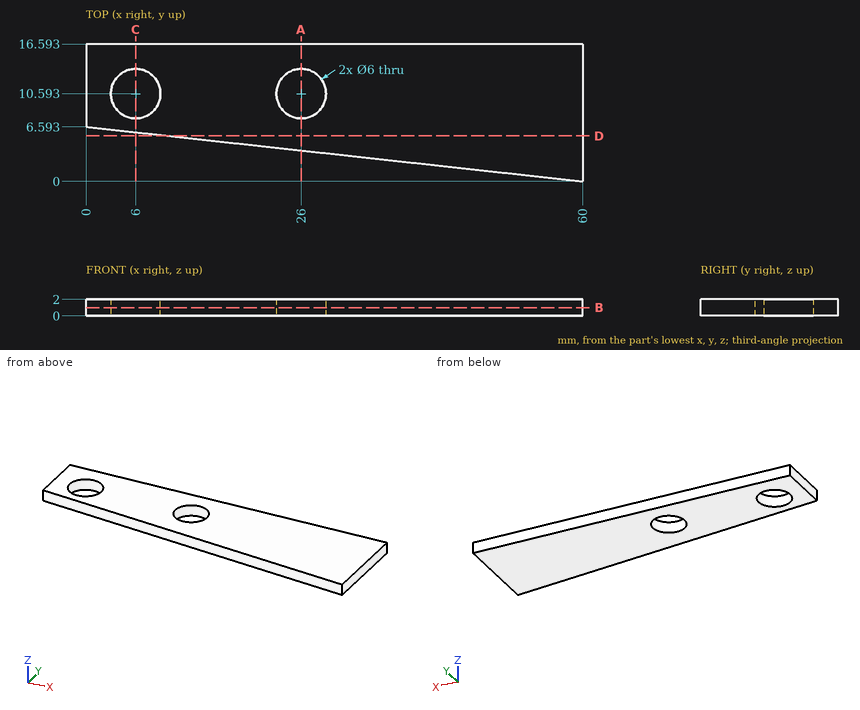
Here's the drawing with two shaded views (mm, measured from the low corner). I have some questions. Coordinates: 2 decimals unless noted, no trailing zeros. Loops run counter-clockwise (first coordinate to the right, second up) from the corner with the lowest first, then second, coordinate; pieces in that order, holes last. Notation, with made-up numbers: (0.25, 52) -> (41.25, 52) arc R17 cw to (41.25, 80) -> close; hole circle Ø8 at (60.25, 75.25). An arc over 180 degrees is marked (long way). Use one line per item in the form item = value. Start each with the question number.
(1) Will these pins go through, and if not, where does the flat tip stop? pin 1 (5.5 mm diameter, centred on x = 26, y = 10.59, fed in from +Z); pin 2 (4 mm diameter, centred on x = 51.5, y = 7, fed in from -Z).
(2) If we section it at A-A (x = 26): Please give me the cut outline in (y, z).
(3) If we section it at C-C (x = 6): Please give me the cut outline in (y, z).
(4) If we section it at B-B (z = 1): Please give me the cut outline in (x, y).
(5) If we section it at D-D (y = 5.5): Please give me the cut outline in (x, z), then the cut area to 3 significant figures.
(6) Please list where these lines run through material, in increasing order: line 1 along X through (y, z) = (12.5, 0.1) (1 decimal); line 2 along X through (y, z) = (10, 1.3); line 3 along Y through (x, z) = (25.5, 0.7) (1 decimal).
Verdict:
q1.pin_1 = through
q1.pin_2 = 0
q2.outline = (3.74, 0) -> (7.59, 0) -> (7.59, 2) -> (3.74, 2) -> close; (13.59, 0) -> (16.59, 0) -> (16.59, 2) -> (13.59, 2) -> close
q3.outline = (5.93, 0) -> (7.59, 0) -> (7.59, 2) -> (5.93, 2) -> close; (13.59, 0) -> (16.59, 0) -> (16.59, 2) -> (13.59, 2) -> close
q4.outline = (0, 6.59) -> (60, 0) -> (60, 16.59) -> (0, 16.59) -> close; hole circle Ø6 at (6, 10.59); hole circle Ø6 at (26, 10.59)
q5.outline = (9.95, 0) -> (60, 0) -> (60, 2) -> (9.95, 2) -> close
q5.area = 100 mm²
q6.line_1 = 0 to 3.7, 8.3 to 23.7, 28.3 to 60
q6.line_2 = 0 to 3.06, 8.94 to 23.06, 28.94 to 60
q6.line_3 = 3.8 to 7.6, 13.6 to 16.6
